Could you check a few things on this model? Use its own coordinates, in mm. Round coordinates to 2 decimals unless told otherwise and drop trailing zeros. Write each loop counter-clockwise with the first axis right and the second up, starting at its lowest first coordinate (ties: lowest second). Pieces come first, ordered by that corner, then holes. Notation, with made-up numbers: (4.25, -15) -> (63.25, -15) arc R26 ccw to (63.25, 22) -> close; hole circle Ø2 at (2, 38). An arc over 180 degrees is marked (long way). Answer as CSV lines item,"result". Start each with the question number.
Q1. Imagine slicing it at A-A on y = 482. Please give me the cut outline in (x, z) (3 decimals).
Q2. If I drill on line 1 (Z direction, x = -10.2, y = 1060.45); line 2 (Y direction, x = 11.25, z = -6.35); line 3 (Z direction, x = -0.25, y = 421) (3 decimals), over which ranges is the centre line in solid material (lowest first)? Write a range as [from, to].
Q3. Will these pins go through, and if not, where does the flat tip stop? pin 1 Ø10 at (x, z) = (-8, 9.5) entering from +Y; pin 2 Ø1.9 at (y, z) = (1111.25, 6.35) entering from +X.
from build123d import *

# Parameters (mm, degrees)
SKETCH1_W                    = 25.4
SKETCH1_H                    = 25.4
SKETCH1_W_2                  = 19.05
SKETCH1_H_2                  = 19.05
BOSS_EXTRUDE1_DEPTH          = 1117.6
CUT_EXTRUDE1_REACH           = 1119.961
SKETCH2_W                    = 19.05
SKETCH2_H                    = 25.4
F_3_8_CLEARANCE_HOLE1_D      = 10.0838
F_10_CLEARANCE_HOLE1_REACH   = 1502.875
F_10_CLEARANCE_HOLE1_BORE_R  = 2.5527
F_1_8_0_125_DIAMETER_HOLE1_D = 3.175
F_10_CLEARANCE_HOLE2_D       = 5.1054


with BuildPart() as part:
    # Sketch1 → Boss-Extrude1 (new body)
    with BuildSketch(Plane(origin=(0, 0, 0), x_dir=(1, 0, 0), z_dir=(0, 1, 0))):
        Rectangle(SKETCH1_W, SKETCH1_H)
        Rectangle(SKETCH1_W_2, SKETCH1_H_2, mode=Mode.SUBTRACT)
    extrude(amount=BOSS_EXTRUDE1_DEPTH)

    # Sketch2 → Cut-Extrude1 (cut, up to next)
    with BuildSketch(Plane(origin=(12.7, 0, 0), x_dir=(0, 0, -1), z_dir=(1, 0, 0)), mode=Mode.PRIVATE) as cut_extrude1_sk1:
        with Locations((0, 1079.5)):
            Rectangle(SKETCH2_W, SKETCH2_H)
    cut_extrude1_tool1 = extrude(cut_extrude1_sk1.sketch, amount=-CUT_EXTRUDE1_REACH, mode=Mode.PRIVATE) & part.part
    add(cut_extrude1_tool1.solids().sort_by_distance((12.7, 1079.5, 0))[0], mode=Mode.SUBTRACT)

    # 3/8 Clearance Hole1 (through all)
    with Locations(Plane.XY.offset(12.7)):
        with Locations((6.35, 1079.5)):
            Hole(F_3_8_CLEARANCE_HOLE1_D / 2)

    # #10 Clearance Hole1 bore → #10 Clearance Hole1 (cut, up to next)
    with BuildSketch(Plane(origin=(-12.7, -56.379087674, -922.047250894), x_dir=(0, 0, 1), z_dir=(-1, 0, 0)), mode=Mode.PRIVATE) as f_10_clearance_hole1_sk1:
        with Locations((922.047250894, 138.929087674)):
            Circle(F_10_CLEARANCE_HOLE1_BORE_R)
    f_10_clearance_hole1_tool1 = extrude(f_10_clearance_hole1_sk1.sketch, amount=-F_10_CLEARANCE_HOLE1_REACH, mode=Mode.PRIVATE) & part.part
    # #10 Clearance Hole1 bore → #10 Clearance Hole1 (cut, up to next)
    with BuildSketch(Plane(origin=(-12.7, -56.379087674, -922.047250894), x_dir=(0, 0, 1), z_dir=(-1, 0, 0)), mode=Mode.PRIVATE) as f_10_clearance_hole1_sk2:
        with Locations((922.047250894, 113.529087674)):
            Circle(F_10_CLEARANCE_HOLE1_BORE_R)
    f_10_clearance_hole1_tool2 = extrude(f_10_clearance_hole1_sk2.sketch, amount=-F_10_CLEARANCE_HOLE1_REACH, mode=Mode.PRIVATE) & part.part
    # #10 Clearance Hole1 bore → #10 Clearance Hole1 (cut, up to next)
    with BuildSketch(Plane(origin=(-12.7, -56.379087674, -922.047250894), x_dir=(0, 0, 1), z_dir=(-1, 0, 0)), mode=Mode.PRIVATE) as f_10_clearance_hole1_sk3:
        with Locations((922.047250894, 69.079087674)):
            Circle(F_10_CLEARANCE_HOLE1_BORE_R)
    f_10_clearance_hole1_tool3 = extrude(f_10_clearance_hole1_sk3.sketch, amount=-F_10_CLEARANCE_HOLE1_REACH, mode=Mode.PRIVATE) & part.part
    add(f_10_clearance_hole1_tool1.solids().sort_by_distance((-12.7, 82.55, 0))[0], mode=Mode.SUBTRACT)
    add(f_10_clearance_hole1_tool2.solids().sort_by_distance((-12.7, 57.15, 0))[0], mode=Mode.SUBTRACT)
    add(f_10_clearance_hole1_tool3.solids().sort_by_distance((-12.7, 12.7, 0))[0], mode=Mode.SUBTRACT)

    # 1/8 (0.125) Diameter Hole1 (through all)
    with Locations(Plane(origin=(12.7, 0, 0), x_dir=(0, 0, -1), z_dir=(1, 0, 0))):
        with Locations((6.35, 1060.45), (6.35, 1098.55), (-6.35, 1111.25), (-6.35, 1098.55), (6.35, 1111.25), (-6.35, 1060.45)):
            Hole(F_1_8_0_125_DIAMETER_HOLE1_D / 2)

    # #10 Clearance Hole2 (through all)
    with Locations(Plane.XY.offset(12.7)):
        with Locations((112.944997341, 382.363477044), (-5.55625, 6.35), (-5.55625, 34.925), (-5.55625, 92.075), (-5.55625, 63.5)):
            Hole(F_10_CLEARANCE_HOLE2_D / 2)


solid = part.part
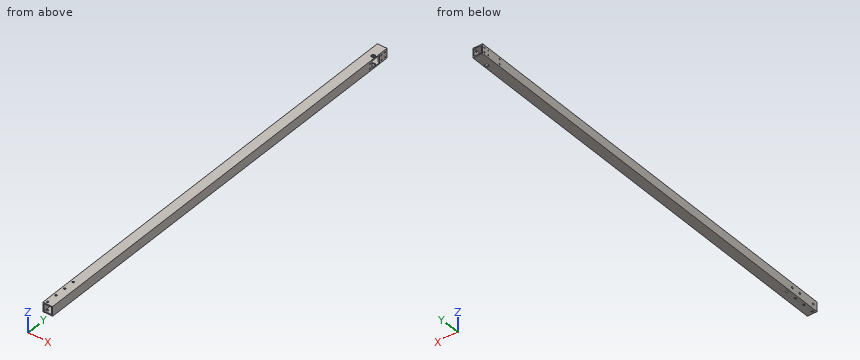
Checks:
1,outline,"(-12.7, -12.7) -> (12.7, -12.7) -> (12.7, 12.7) -> (-12.7, 12.7) -> close; hole (-9.525, -9.525) -> (9.525, -9.525) -> (9.525, 9.525) -> (-9.525, 9.525) -> close"
2,line 1,"[-12.7, -7.94], [-4.76, 4.76], [7.94, 12.7]"
2,line 2,"[0, 1058.86], [1062.04, 1066.8], [1092.2, 1096.96], [1100.14, 1109.66], [1112.84, 1117.6]"
2,line 3,"[-12.7, -9.525], [9.525, 12.7]"
3,pin 1,"y = 1117.6"
3,pin 2,"through"
